For this review, take the finished solid that the model builds, in its own axes (mm). A direction names the side the tool comes from. Give positions to 0.01 mm unless a question says otherwise; leave off trailing zeros. Write each loop counter-clockwise with the first axis right and the second up, starting at its lowest first coordinate (ties: lowest second). Pieces come first, ordered by that corner, then holes. Notation, with made-up numbers: (55.5, 80.5) -> (59.5, 80.5) arc R17 ccw to (59.5, 92.5) -> close; hole circle Ø11 at (9, 14). An arc over 180 degrees is marked (long way). Answer as CSV lines item,"result".
```python
from build123d import *

# Parameters (mm, degrees)
F0_W          = 570
F0_H          = 40
F1_DEPTH      = 40
F0_W_2        = 40
F0_H_2        = 570
F2_DEPTH      = 760
F2_DEPTH_BACK = 145
F3_W          = 5
F3_H          = 35
F3_H_2        = 5
F3_W_2        = 35
F4_DEPTH      = 40
F5_DEPTH      = 240


with BuildPart() as f1:
    # F0 (on Top) → F1 (new body)
    with BuildSketch(Plane.XY):
        with Locations((0, 305)):
            Rectangle(F0_W, F0_H)
    extrude(amount=-F1_DEPTH)



with BuildPart() as f1b:
    # F0 (on Top) → F1, piece 2 (new body)
    with BuildSketch(Plane.XY):
        with Locations((-305, 0)):
            Rectangle(F0_W_2, F0_H_2)
    extrude(amount=-F1_DEPTH)


with BuildPart() as f1c:
    # F0 (on Top) → F1, piece 3 (new body)
    with BuildSketch(Plane.XY):
        with Locations((305, 0)):
            Rectangle(F0_W_2, F0_H_2)
    extrude(amount=-F1_DEPTH)


with BuildPart() as f1d:
    # F0 (on Top) → F1, piece 4 (new body)
    with BuildSketch(Plane.XY):
        with Locations((0, -305)):
            Rectangle(F0_W, F0_H)
    extrude(amount=-F1_DEPTH)


with BuildPart() as f1_1:
    add(f1.part)

    add(f1b.part)  # F2 merges F1b

    add(f1c.part)  # F2 merges F1c

    add(f1d.part)  # F2 merges F1d
    # F0 (on Top) → F2 (join, two sides)
    with BuildSketch(Plane.XY) as f2_sk:
        with Locations((-305, 305)):
            Rectangle(F0_W_2, F0_H)
        with Locations((305, 305)):
            Rectangle(F0_W_2, F0_H)
        with Locations((305, -305)):
            Rectangle(F0_W_2, F0_H)
        with Locations((-305, -305)):
            Rectangle(F0_W_2, F0_H)
    extrude(amount=F2_DEPTH)
    extrude(f2_sk.sketch, amount=-F2_DEPTH_BACK)

    # F3 (on face) → F4 (join)
    with BuildSketch(Plane.XY.offset(760)):
        Polygon((280, 320), (280, 325), (-280, 325), (-280, 320), (-280, 285), (280, 285), align=None)
        with Locations((-282.5, 302.5)):
            Rectangle(F3_W, F3_H)
        with Locations((-282.5, 322.5)):
            Rectangle(F3_W, F3_H_2)
        with Locations((-302.5, 282.5)):
            Rectangle(F3_W_2, F3_H_2)
        with Locations((-322.5, 282.5)):
            Rectangle(F3_W, F3_H_2)
        Polygon((-285, -280), (-285, 280), (-320, 280), (-325, 280), (-325, -280), (-320, -280), align=None)
        with Locations((282.5, 302.5)):
            Rectangle(F3_W, F3_H)
        with Locations((282.5, 322.5)):
            Rectangle(F3_W, F3_H_2)
        with Locations((302.5, 282.5)):
            Rectangle(F3_W_2, F3_H_2)
        with Locations((322.5, 282.5)):
            Rectangle(F3_W, F3_H_2)
        Polygon((325, -280), (325, 280), (320, 280), (285, 280), (285, -280), (320, -280), align=None)
        with Locations((302.5, -282.5)):
            Rectangle(F3_W_2, F3_H_2)
        with Locations((322.5, -282.5)):
            Rectangle(F3_W, F3_H_2)
        with Locations((282.5, -302.5)):
            Rectangle(F3_W, F3_H)
        with Locations((282.5, -322.5)):
            Rectangle(F3_W, F3_H_2)
        Polygon((280, -320), (280, -285), (-280, -285), (-280, -320), (-280, -325), (280, -325), align=None)
        with Locations((-282.5, -302.5)):
            Rectangle(F3_W, F3_H)
        with Locations((-282.5, -322.5)):
            Rectangle(F3_W, F3_H_2)
        with Locations((-302.5, -282.5)):
            Rectangle(F3_W_2, F3_H_2)
        with Locations((-322.5, -282.5)):
            Rectangle(F3_W, F3_H_2)
    extrude(amount=-F4_DEPTH)

    # F3 (on face) → F5 (join)
    with BuildSketch(Plane.XY.offset(760)):
        with Locations((302.5, -282.5)):
            Rectangle(F3_W_2, F3_H_2)
        with Locations((302.5, -302.5)):
            Rectangle(F3_W_2, F3_H)
        with Locations((282.5, -302.5)):
            Rectangle(F3_W, F3_H)
        with Locations((282.5, -282.5)):
            Rectangle(F3_W, F3_H_2)
        with Locations((302.5, 302.5)):
            Rectangle(F3_W_2, F3_H)
        with Locations((302.5, 282.5)):
            Rectangle(F3_W_2, F3_H_2)
        with Locations((282.5, 282.5)):
            Rectangle(F3_W, F3_H_2)
        with Locations((282.5, 302.5)):
            Rectangle(F3_W, F3_H)
        with Locations((-302.5, -302.5)):
            Rectangle(F3_W_2, F3_H)
        with Locations((-302.5, -282.5)):
            Rectangle(F3_W_2, F3_H_2)
        with Locations((-282.5, -282.5)):
            Rectangle(F3_W, F3_H_2)
        with Locations((-282.5, -302.5)):
            Rectangle(F3_W, F3_H)
    extrude(amount=F5_DEPTH)


solid = f1_1.part
```
Q1. Add section B-B (x = 67.5). Write out the cut boundary in (y, z), plus the area to 3 significant figures.
Answer block:
outline,"(-325, -40) -> (-285, -40) -> (-285, 0) -> (-325, 0) -> close; (-325, 720) -> (-285, 720) -> (-285, 760) -> (-325, 760) -> close; (285, -40) -> (325, -40) -> (325, 0) -> (285, 0) -> close; (285, 720) -> (325, 720) -> (325, 760) -> (285, 760) -> close"
area,"6,400 mm2"
Q2. Add section A-A (z = 615). Write out the cut boundary in (x, y), plus the area to 3 significant figures.
Answer block:
outline,"(-325, -325) -> (-285, -325) -> (-285, -285) -> (-325, -285) -> close; (-325, 285) -> (-285, 285) -> (-285, 325) -> (-325, 325) -> close; (285, -325) -> (325, -325) -> (325, -285) -> (285, -285) -> close; (285, 285) -> (325, 285) -> (325, 325) -> (285, 325) -> close"
area,"6,400 mm2"
Q3. For faces 4 (the flat face through (-280, -300, 878)), 5 (the flat face through (305, 285, -92)), 6 (the flat face through (285, 305, 355)), 7 (the flat face through (-285, -4, -20)), list the 3-axis set-ups (+Z, -Z, +X, -X, +Y, -Y) from which the entire face can be reached by the end or side of a thin tool; tool diameter is ignored.
Answer block:
face 4,"+Z, +Y, -Y"
face 5,"-Z, +X, -X"
face 6,"+Y, -Y"
face 7,"+Z, -Z"
Q4. Add section C-C (z = 816). Write out the cut boundary in (x, y), plus the area to 3 significant figures.
Answer block:
outline,"(-320, -320) -> (-280, -320) -> (-280, -280) -> (-320, -280) -> close; (280, -320) -> (320, -320) -> (320, -280) -> (280, -280) -> close; (280, 280) -> (320, 280) -> (320, 320) -> (280, 320) -> close"
area,"4,800 mm2"
Q5. Clearance check with flat-ended pins moving along their axes: pin 1 (5.5 mm diameter, centred on x = -283, y = -282.5, fed in from -Z); pin 2 (20 mm diameter, centred on x = -295, z = 894.5, fed in from -Y); pin 3 (12 mm diameter, centred on x = 292.5, z = 899, fed in from +Y). State where each tip first meets the part, or that it passes through.
Answer block:
pin 1,"stops at z = -40"
pin 2,"stops at y = -320"
pin 3,"stops at y = 320"
Q6. Draft analysis for pull direction Y (two halves, no side actions). For faces 1 (the flat face through (305, -305, -145)), 2 (the flat face through (300, 320, 878)), 3 (the flat face through (-305, 4, 720)), state which applies: released by +Y, released by -Y, zero draft, split by the parting line, or undercut.
Answer block:
face 1,"zero draft"
face 2,"released by +Y"
face 3,"undercut"
